Study the drawing (mm; zero at the part's minimum x, y, z) and answer. Give positions to 0.01 mm unless a question says otherwise; leave off trailing zeros. Loops run counter-clockwise (first coordinate to the right, second up) from the corner with the lowest first, then second, coordinate; pieces in that order, holes last. Notation, with made-up numbers: (69, -40) - (112, -40) arc R23 cw to (112, -15) - close; hole circle Ø10 at (75, -0.75). An arc over 180 degrees is marked (long way). Write item = value, one per line. Start each with the question number.
1) The mould has two halves that part along Y. Classify the marked faces 1, 2, 3 and 4: +Y half, -Y half, draft (parallel to the pull), parting line (faces both ways), or undercut.
2) Consider probe 1 along Y at (x, z) = (23.5, 18.75) (1 decimal); probe 2 along Y at (x, z) = (26, 2.75); probe 3 along X at (y, z) = (35.5, 6.25) (1 decimal). Determine where each line is inside the solid, lowest interval first.
3) The part is cut by section A-A on x = 26. Write down the section's boundary in (y, z).
4) The part is cut by section C-C on y = 57.5. Write down the section's boundary in (x, z).
5) The part is cut by section D-D on y = 30. Write down the section's boundary in (x, z) (1 decimal).
6) The part is cut by section B-B on z = 4. Write down the section's boundary in (x, y).
7) Flat-ended cylindrical pins translate along their axes: P1, Ø2, axis at y = 58.5, z = 13.5, coming from the -X side (1 decimal); P2, Ø12, axis at y = 48.5, z = 7, coming from the -X side (1 decimal). Find the tip coordinate at first contact, or state that the pin passes through.
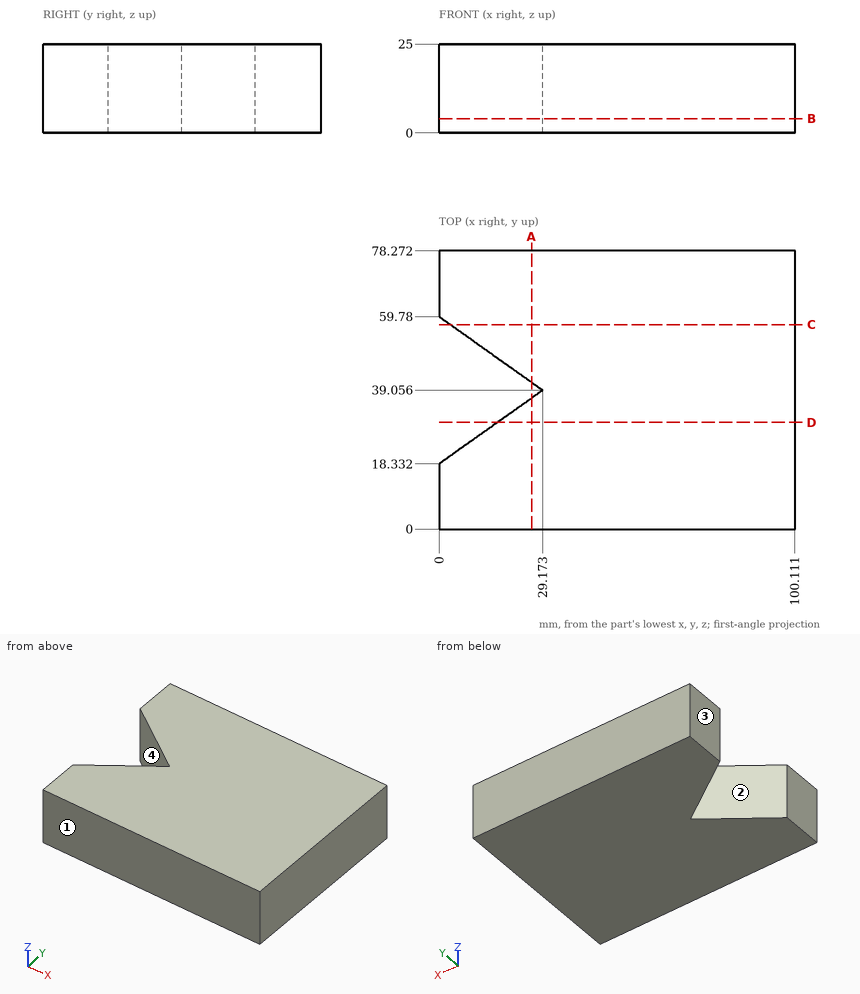
Answer below:
q1.face_1 = -Y half
q1.face_2 = undercut
q1.face_3 = draft
q1.face_4 = undercut
q2.probe_1 = 0 to 35, 43.1 to 78.3
q2.probe_2 = 0 to 36.8, 41.31 to 78.27
q2.probe_3 = 24.2 to 100.1
q3.outline = (0, 0) - (36.8, 0) - (36.8, 25) - (0, 25) - close; (41.31, 0) - (78.27, 0) - (78.27, 25) - (41.31, 25) - close
q4.outline = (3.21, 0) - (100.11, 0) - (100.11, 25) - (3.21, 25) - close
q5.outline = (16.4, 0) - (100.1, 0) - (100.1, 25) - (16.4, 25) - close
q6.outline = (0, 0) - (100.11, 0) - (100.11, 78.27) - (0, 78.27) - (0, 59.78) - (29.17, 39.06) - (0, 18.33) - close
q7.P1 = 0.4
q7.P2 = 7.4
